Input: dimensioned drawing with shaded views. Units: mm. Origin: part minimum x, y, z. A direction names the side the tool comes from. Give positions to 0.01 mm unless a question says otherwise; leave off trailing zeros. Loops run counter-clockwise (first coordinate to the right, second up) from the corner with the lowest first, then second, coordinate; pieces in that order, holes last.
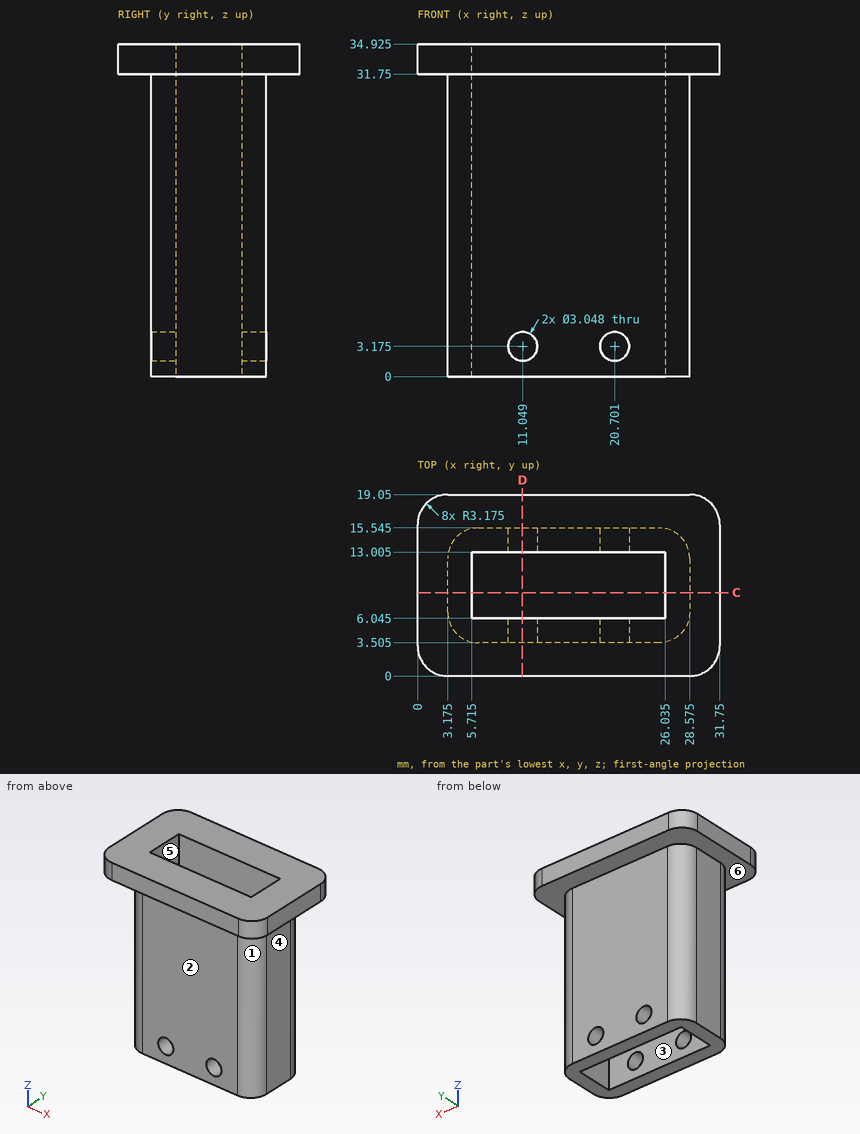
(1) Reachability of the marked faces 1, 2 and 3 from +Z, -Z, +X, -X, +Y, -Y: full face, straight path, thin tool, end or side. Return the list, or none.
A:
face 1: -Z, +X, -Y
face 2: -Z, +X, -X, -Y
face 3: +Z, -Z
(2) First-contact query: pin 1 (4.5 mm diameter, centred on y = 10, z = 12, fed in from +X) (3 decimals); pin 2 (9.5 mm diameter, centred on x = 14, z = 21, fed in from -Y) (3 decimals); pin 3 (15 mm diameter, centred on x = 20.5, z = 9, fed in from +Y) (3 decimals); pin 4 (4 mm diameter, centred on x = 14, y = 7, fed in from +Z) (3 decimals). Flat tips, straight axial feed; report the tip coordinate or a pass-through.
A:
pin 1: stops at x = 28.575
pin 2: stops at y = 3.505
pin 3: stops at y = 15.545
pin 4: stops at z = 34.925
(3) Section C-C, the plane y = 8.75. Return the cut outline in (x, z) (3 decimals).
A:
outline: (0, 31.75) - (3.175, 31.75) - (3.175, 0) - (5.715, 0) - (5.715, 34.925) - (0, 34.925) - close; (26.035, 0) - (28.575, 0) - (28.575, 31.75) - (31.75, 31.75) - (31.75, 34.925) - (26.035, 34.925) - close
(4) Section D-D, the plane x = 11. Count the separate pieces of the cut face and the enclosed holes in it, then the cut area to 3 significant figures.
A:
separate pieces: 4
enclosed holes: 0
area: 184 mm2
(5) Ray query, line 1 along Y through (x, z) = (16.5, 18) (1 decimal); line 2 along X through (y, z) = (8.75, 26.5) (3 decimals); line 3 along Z through (x, y) = (30.5, 12.5) (3 decimals). Return the intervals inside material, ascending.
A:
line 1: y = 3.5 to 6, 13 to 15.5
line 2: x = 3.175 to 5.715, 26.035 to 28.575
line 3: z = 31.75 to 34.925
(6) Mould query, pull axis X, two halves, no side actions, for the marked faces 4, 5 and 6. Classes: pulls with the +X half, pulls with the -X half, needs draft (parallel to the pull), parting line crosses it, or undercut.
A:
face 4: pulls with the +X half
face 5: undercut
face 6: needs draft
